The figure shows three views and two pictorial views of one solid part (mm, origin at its lowest corner). Answer the questions. A direction names the side the tool comes from. Coordinates: 2 decimals unless noted, no trailing zeros. Write each loop counter-clockwise with the first axis right and the second up, starting at its lowest first coordinate (ties: lowest second). Pieces come first, ordered by that corner, then holes. Notation, with made-up numbers: M 27,21 L 82,21 A28 cw 82,40 Z; hole C -38.5,85 d11. An arc over 180 degrees is marked long. Answer as CSV lines item,"result".
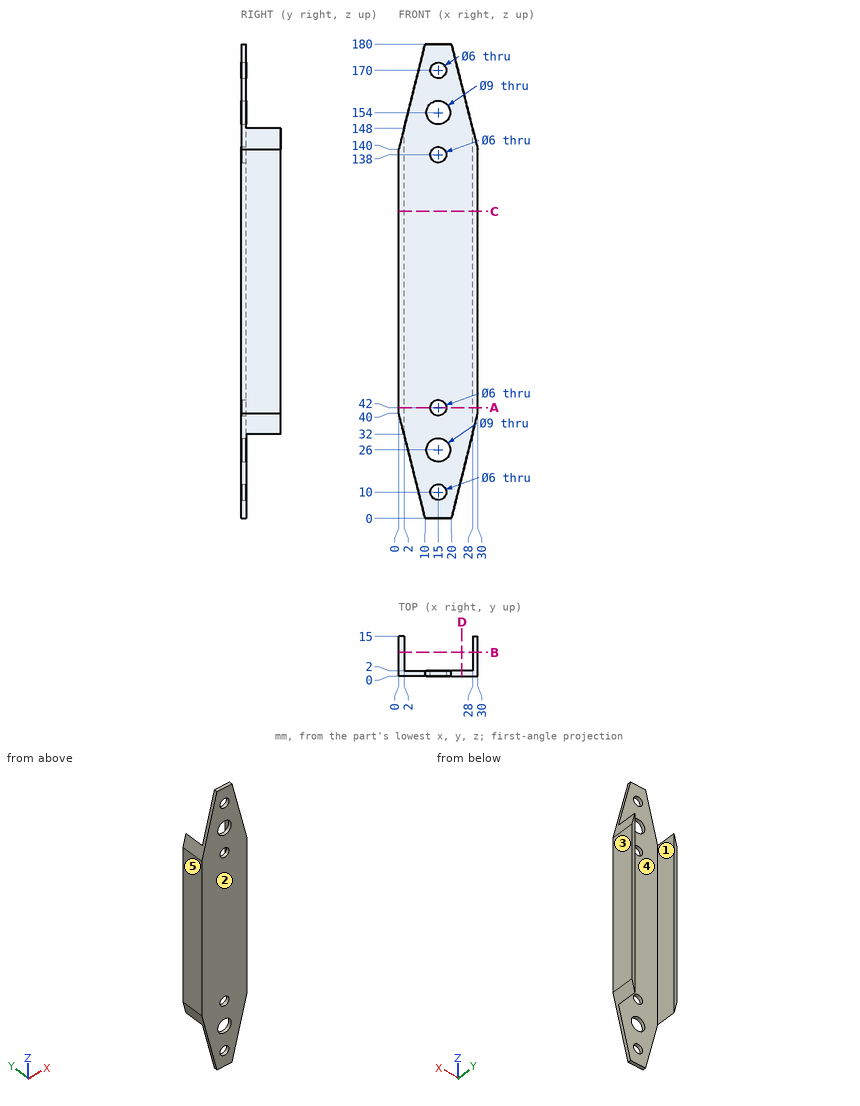
Q1. The mould has two halves that part along X. Classify the marked faces 3, 4 and 5: pulls with the +X half, pulls with the -X half, needs draft (parallel to the pull), parting line crosses it, or undercut.
Output:
face 3,"pulls with the +X half"
face 4,"undercut"
face 5,"pulls with the -X half"
Q2. Find section B-B (y = 9). Give the vertices of the cut face in (x, z), and give its area (3 significant figures).
Output:
outline,"M 0,40 L 2,32 L 2,148 L 0,140 Z; M 28,32 L 30,40 L 30,140 L 28,148 Z"
area,"432 mm2"
Q3. For the marked faces 1 and 2, determine the directions among +Z, -Z, +X, -X, +Y, -Y from which every point of the face is accessible in a straight line to the end or side of a thin tool.
Output:
face 1,"+Z, -Z, +Y"
face 2,"+Z, -Z, +X, -X, -Y"
Q4. Find section C-C (z = 116.5). Give the vertices of the cut face in (x, y).
Output:
outline,"M 0,0 L 30,0 L 30,15 L 28,15 L 28,2 L 2,2 L 2,15 L 0,15 Z"
Q5. Flat-ended cylindrical pins translate along their axes: pin 1 Ø8 at (x, z) = (15, 10) entering from +Y; pin 2 Ø3 at (y, z) = (2, 160.5) entering from +X; pin 3 Ø1.5 at (y, z) = (1.5, 33) entering from +X. Find the tip coordinate at first contact, or state that the pin passes through.
Output:
pin 1,"y = 2"
pin 2,"x = 25.25"
pin 3,"x = 28.44"
Q6. Straight lines are drawn through the part: line 1 (X direction, y = 4, z = 42); line 2 (X direction, y = 1.45, z = 42); line 3 (Y direction, x = 3.5, z = 73.5). For each, find the intervals that lie inside material, in ascending order.
Output:
line 1,"0 to 2, 28 to 30"
line 2,"0 to 12, 18 to 30"
line 3,"0 to 2"
Q7. Find section D-D (x = 24). Give the vertices of the cut face in (y, z).
Output:
outline,"M 0,16 L 2,16 L 2,164 L 0,164 Z"
Q8. Find section A-A (z = 42). Give the vertices of the cut face in (x, y).
Output:
outline,"M 0,0 L 12,0 L 12,2 L 2,2 L 2,15 L 0,15 Z; M 18,0 L 30,0 L 30,15 L 28,15 L 28,2 L 18,2 Z"
